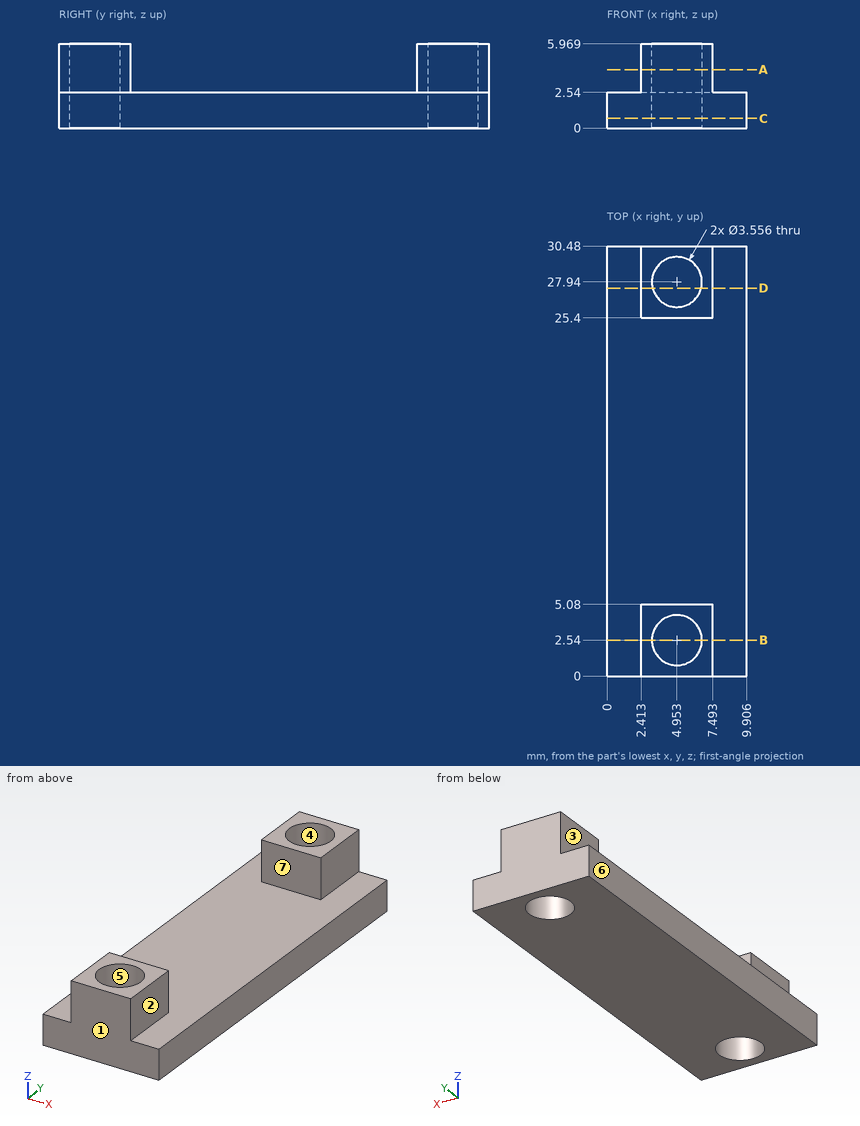
Can you work these out from the drawing? Everything is in mm from the part's minimum corner. A direction names the side the tool comes from. Coordinates: 2 decimals unless noted, no trailing zeros. Loops run counter-clockwise (first coordinate to the right, second up) from the corner with the lowest first, then second, coordinate; pieces in that order, holes last. Notation, with made-up numbers: (-1.75, 52) -> (39.25, 52) arc R9 ccw to (39.25, 69) -> close; hole circle Ø7 at (55.25, 68.5). An arc over 180 degrees is marked (long way). Return JSON: item names as keys, results as strings.
1) For the marked faces 1, 2 and 3, which set-ups out of +Z, -Z, +X, -X, +Y, -Y let a thin tool reach every point of the face, with its end or its side?
Results below:
{"face 1": "+Z, -Z, +X, -X, -Y", "face 2": "+Z, +X, +Y, -Y", "face 3": "+Z, -X, +Y, -Y"}
2) If we section it at A-A, the plane z = 4.15: Write out the boundary of the cut face in (x, y), then the cut area to 3 significant figures.
Results below:
{"outline": "(2.41, 0) -> (7.49, 0) -> (7.49, 5.08) -> (2.41, 5.08) -> close; (2.41, 25.4) -> (7.49, 25.4) -> (7.49, 30.48) -> (2.41, 30.48) -> close; hole circle Ø3.56 at (4.95, 2.54); hole circle Ø3.56 at (4.95, 27.94)", "area": "31.7 mm²"}
3) I need wall thicknesses on line 1 (Y direction, x = 2.5, z = 2.8); line 2 (Y direction, x = 5.25, z = 5.5); line 3 (X direction, y = 28, z = 3.75). Which ranges of each line are inside material? Lowest first, please. Write a range as from..to.
Results below:
{"line 1": "0..5.08, 25.4..30.48", "line 2": "0..0.79, 4.29..5.08, 25.4..26.19, 29.69..30.48", "line 3": "2.41..3.18, 6.73..7.49"}
4) If we section it at B-B, the plane y = 2.54: Write out the boundary of the cut face in (x, z) (3 decimals), then the cut area to 3 significant figures.
Results below:
{"outline": "(0, 0) -> (3.175, 0) -> (3.175, 5.969) -> (2.413, 5.969) -> (2.413, 2.54) -> (0, 2.54) -> close; (6.731, 0) -> (9.906, 0) -> (9.906, 2.54) -> (7.493, 2.54) -> (7.493, 5.969) -> (6.731, 5.969) -> close", "area": "21.4 mm²"}
5) If we section it at D-D, the plane y = 27.5: Write out the boundary of the cut face in (x, z).
Results below:
{"outline": "(0, 0) -> (3.23, 0) -> (3.23, 5.97) -> (2.41, 5.97) -> (2.41, 2.54) -> (0, 2.54) -> close; (6.68, 0) -> (9.91, 0) -> (9.91, 2.54) -> (7.49, 2.54) -> (7.49, 5.97) -> (6.68, 5.97) -> close"}
6) If we section it at C-C, the plane z = 0.7: Write out the boundary of the cut face in (x, y), then the cut area to 3 significant figures.
Results below:
{"outline": "(0, 0) -> (9.91, 0) -> (9.91, 30.48) -> (0, 30.48) -> close; hole circle Ø3.56 at (4.95, 2.54); hole circle Ø3.56 at (4.95, 27.94)", "area": "282 mm²"}
7) Thinking about a two-plate mould opening in X: for the marked faces 4, 5, 6 and 7, which applies, +X half, -X half, draft (parallel to the pull), parting line (faces both ways), or undercut?
Results below:
{"face 4": "undercut", "face 5": "undercut", "face 6": "-X half", "face 7": "draft"}
8) Will these pins go through, and if not, where does the flat tip stop? pin 1 (1 mm diameter, centred on y = 27, z = 4, fed in from +X); pin 2 (1 mm diameter, centred on y = 27, z = 4, fed in from -X); pin 3 (5 mm diameter, centred on x = 5, y = 11.5, fed in from -Z); pin 4 (4 mm diameter, centred on x = 8, y = 11, fed in from +Z).
Results below:
{"pin 1": "x = 7.49", "pin 2": "x = 2.41", "pin 3": "z = 0", "pin 4": "z = 2.54"}
